```python
from build123d import *

# Parameters (mm, degrees)
F0_R     = 14.79582
F1_DEPTH = 25.4
F2_T     = -2.54
F3_W     = 17.056221
F3_H     = 33.380184
F4_DEPTH = 174.498


with BuildPart() as f1:
    # F0 (on Front) → F1 (new body)
    with BuildSketch(Plane.XZ):
        with Locations((-10.001251, 5.218043)):
            Circle(F0_R)
    extrude(amount=F1_DEPTH)

    # F2
    f2_openings = [f1.faces().sort_by_distance(p)[0] for p in [
        (-10.001251, -25.4, 5.218043),
    ]]
    offset(amount=F2_T, openings=f2_openings)

    # F3 (on Front) → F4 (join)
    with BuildSketch(Plane.XZ):
        with Locations((-9.636964, 14.683178)):
            Rectangle(F3_W, F3_H)
    extrude(amount=-F4_DEPTH)


solid = f1.part
```
Verification items for the finished model (mm, model axes). A direction names the side the tool comes from. Give positions to 0.01 mm unless a question says otherwise; leave off trailing zeros. Order: outer loops, then holes, each group sorted by start corner. A loop starts at its lowest first (then second) coordinate and runs counter-clockwise, first axis right, second up. Notation, with made-up numbers: M 87.25,25 L 146.25,25 A24 cw 146.25,55 Z; hole C 18,-35 d5. An arc over 180 degrees is marked long. Return JSON: item names as keys, results as strings. Group by question number.
1) Go/stop test with flat-tipped pins: pin 1 Ø2 at (x, y) = (-9, 67) entering from -Z; pin 2 Ø3 at (y, z) = (14, 24.5) entering from -X; pin 3 Ø1 at (y, z) = (63.5, 26.5) entering from +X. Record where each tip stops, or that it passes through.
2) Section check A-A on z = 25.5. Record the cut outline in (x, y), and give its area (3 significant figures).
3) Scan lines: line 1 (X direction, y = 43, z = -1.5); line 2 (Y direction, x = -6.5, z = 16); line 3 (Z direction, x = -14.75, y = 50). Record each from-to range of solid material in increasing order.
4) Access from +Z, -Z, +X, -X, +Y, -Y to the whole of each face (thin tool, end or side, straight path). Record for faces 5 (the face through (-21, -25.4, 11)), 6 (the face through (-3.174, -12.522, -7.908)), 7 (the face through (-10, 86, -2.007)).
5) Mould release check, pull along X, two halves, no side actions. Record for faces 1 (the face through (-10, 0, -5)), 2 (the face through (-18.165, 86, 14)), 3 (the face through (1.69, -13.81, 8.9)), 4 (the face through (-1.109, 86, 14)): pulls with the +X half, pulls with the -X half, needs draft (parallel to the pull), parting line crosses it, or undercut.
6) Section check C-C on y = 111. Record the cut outline in (x, z), and give its area (3 significant figures).
7) Section check D-D on z = 12. Record the cut outline in (x, y), and give its area (3 significant figures).
8) Section check B-B on x = -5. Record the cut outline in (y, z).
Answer block:
{
 "1": {"pin 1": "stops at z = -2.01", "pin 2": "stops at x = -18.17", "pin 3": "stops at x = -1.11"},
 "2": {"outline": "M -18.17,0 L -1.11,0 L -1.11,174.5 L -18.17,174.5 Z", "area": "2,980 mm^2"},
 "3": {"line 1": "x = -18.17 to -1.11", "line 2": "y = -2.54 to 174.5", "line 3": "z = -2.01 to 31.37"},
 "4": {"face 5": "+Z, -Z, +X, -X, -Y", "face 6": "-Y", "face 7": "-Z, +X, -X, +Y"},
 "5": {"face 1": "needs draft", "face 2": "pulls with the -X half", "face 3": "undercut", "face 4": "pulls with the +X half"},
 "6": {"outline": "M -18.17,-2.01 L -1.11,-2.01 L -1.11,31.37 L -18.17,31.37 Z", "area": "569 mm^2"},
 "7": {"outline": "M -23.15,-25.4 L -20.21,-25.4 L -20.21,-2.54 L 0.21,-2.54 L 0.21,-25.4 L 3.15,-25.4 L 3.15,0 L -1.11,0 L -1.11,174.5 L -18.17,174.5 L -18.17,0 L -23.15,0 Z", "area": "3,180 mm^2"},
 "8": {"outline": "M -25.4,-8.71 L 0,-8.71 L 0,-2.01 L 174.5,-2.01 L 174.5,31.37 L 0,31.37 L 0,19.14 L -25.4,19.14 L -25.4,16.41 L -2.54,16.41 L -2.54,-5.97 L -25.4,-5.97 Z"}
}
